Job drawing, mm, ordinate dimensions from the low corner. One solid piece. Round coordinates to 2 decimals unless told otherwise and drop trailing zeros. Loops run counter-clockwise (first coordinate to the right, second up) from the corner with the lowest first, then second, coordinate; pieces in that order, holes last. Notation, with made-up numbers: (44, 66) - (100, 66) arc R22 cw to (100, 102) - close; hole circle Ø8 at (40, 71.5). An arc over 180 degrees is marked (long way). Answer as CSV lines item,"result". Start each with the question number.
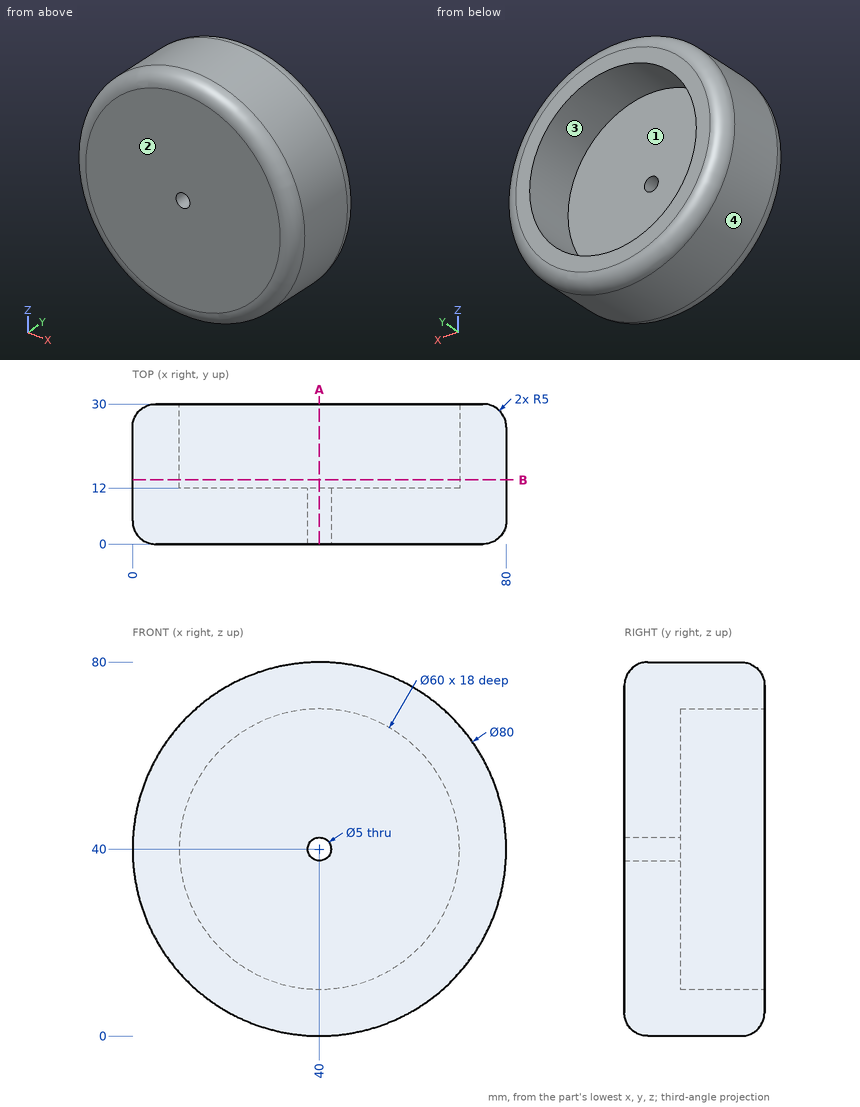
Q1. Band-saw the part on B-B, the plane y = 13.75. List the corners of the cut face in (x, z).
Q2. Wall check: probe 1 along Z at (x, y) = (40, 7.5); probe 2 along Z at (x, y) = (40, 24); probe 3 along X at (y, z) = (24, 61). Give the ranges that are in metal, low to high. Write a range as [from, to].
Q3. Band-saw the part on A-A, the plane x = 40. List the corners of the cut face in (y, z), then the cut area to 3 significant figures.
Q4. Pin check, flat tips, straight feed: pin 1 Ø3 at (y, z) = (13, 12.5) entering from -X; pin 2 Ø12 at (y, z) = (11, 25.5) entering from +X; pin 3 Ø3 at (x, y) = (48, 20.5) entering from -Z. Stop position of each tip, or through.
Q5. Two-plate mould, pull along X, no slides. Class the marked faces 1, 2, 3 and 4: released by +X, released by -X, zero draft, split by the parting line, or undercut.
Reported:
1,outline,"circle Ø80 at (40, 40); hole circle Ø60 at (40, 40)"
2,probe 1,"z = [0, 37.5], [42.5, 80]"
2,probe 2,"z = [0, 10], [70, 80]"
2,probe 3,"x = [5.96, 18.58], [61.42, 74.04]"
3,outline,"(0, 5) arc R5 ccw to (5, 0) - (25, 0) arc R5 ccw to (30, 5) - (30, 10) - (12, 10) - (12, 37.5) - (0, 37.5) - close; (0, 42.5) - (12, 42.5) - (12, 70) - (30, 70) - (30, 75) arc R5 ccw to (25, 80) - (5, 80) arc R5 ccw to (0, 75) - close"
3,area,"1,240 mm2"
4,pin 1,"stops at x = 9.6"
4,pin 2,"stops at x = 79.09"
4,pin 3,"stops at z = 0.53"
5,face 1,"undercut"
5,face 2,"zero draft"
5,face 3,"undercut"
5,face 4,"split by the parting line"
